For this review, use the dimensioned drawing (mm, ordinates from the lowest corner) and the shaded views. A direction names the side the tool comes from. Give positions to 0.01 mm unless a question says otherwise; leave off trailing zeros. Order: outer loops, then holes, each group sorted by start corner. A loop starts at its lowest first (then second) coordinate and runs counter-clockwise, first axis right, second up. Notation, with made-up numbers: (49.25, 55) - (85.25, 55) arc R34 ccw to (85.25, 89) - close; hole circle Ø8 at (63, -25). An arc over 180 degrees is marked (long way). One line per item, written item: value.
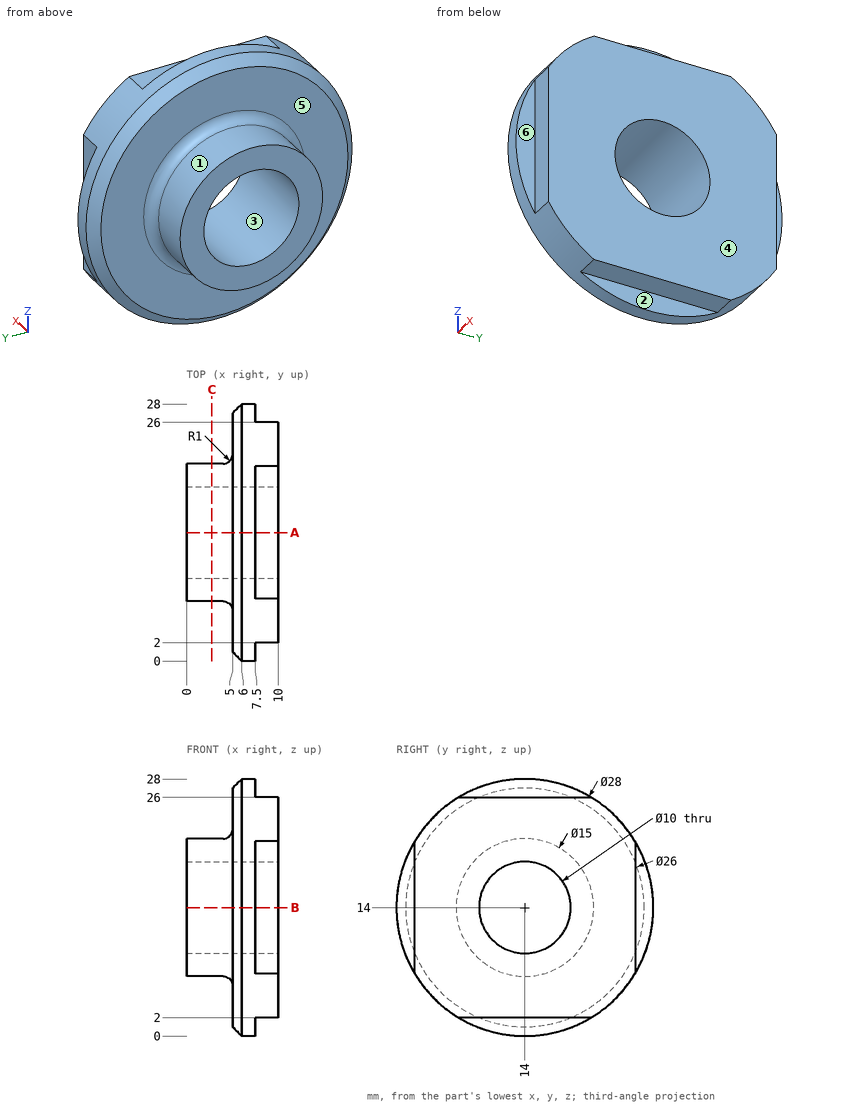
(1) Wall thickness on line 1 (Z direction, x = 3.5, y = 14); line 2 (X direction, y = 8.75, z = 3.5); line 3 (Y direction, x = 9, z = 16.25): over which ranges is each line inside the solid? List them lowest first. Write a range as from..to.
Answers below:
line 1: z = 6.5..9, 19..21.5
line 2: x = 5..10
line 3: y = 2..9.53, 18.47..26
(2) Draft analysis for pull direction Z (two halves, no side actions). For the marked faces 1, 2 and 3, state which applies: pulls with the +Z half, pulls with the -Z half, needs draft (parallel to the pull), parting line crosses it, or undercut.
Answers below:
face 1: parting line crosses it
face 2: needs draft
face 3: undercut
(3) Take a section at C-C (x = 2.75). Write out the cut boundary in (y, z), then the cut area to 3 significant figures.
Answers below:
outline: circle Ø15 at (14, 14); hole circle Ø10 at (14, 14)
area: 98.2 mm^2
(4) Machinability: for the marked faces 4, 5 and 6, which of the approach directions +Z, -Z, +X, -X, +Y, -Y give a long, thin tool a straight path to every point of the face, cutting with its end or side? Answer none if there is none.
Answers below:
face 4: +Z, -Z, +X, +Y, -Y
face 5: -X
face 6: +Z, -Z, +X, -Y
(5) Take a section at A-A (y = 14). Write out the cut boundary in (x, z).
Answers below:
outline: (0, 6.5) - (4, 6.5) arc R1 cw to (5, 5.5) - (5, 1) - (6, 0) - (7.5, 0) - (7.5, 2) - (10, 2) - (10, 9) - (0, 9) - close; (0, 19) - (10, 19) - (10, 26) - (7.5, 26) - (7.5, 28) - (6, 28) - (5, 27) - (5, 22.5) arc R1 cw to (4, 21.5) - (0, 21.5) - close
(6) For P1, Ø2, axis at x = 9, y = 14, coming from the -Z side; P2, Ø2, axis at y = 17.5, z = 0.5, coming from the +X side; P3, Ø0.8, axis at x = 8.5, z = 16, coming from the +Y side, all flat-tipped, find the tip position at first contact; note any pin that passes through.
Answers below:
P1: stops at z = 2
P2: stops at x = 7.5
P3: stops at y = 26
